Source: CAD feature listing. Evaluate the final solid. Frame: model axes, mm. Give positions to 0.01 mm unless a question says otherwise; leave off trailing zeros. Loops run counter-clockwise (first coordinate to the right, second up) from the corner with the lowest first, then second, coordinate; pieces in that order, holes last. Notation, with made-up numbers: (-39, 87) -> (-33, 87) arc R14 cw to (-33, 107) -> close; hole circle Ø6 at (25.25, -40). An arc over 180 degrees is marked (long way). Put each result on its own line as item: value.
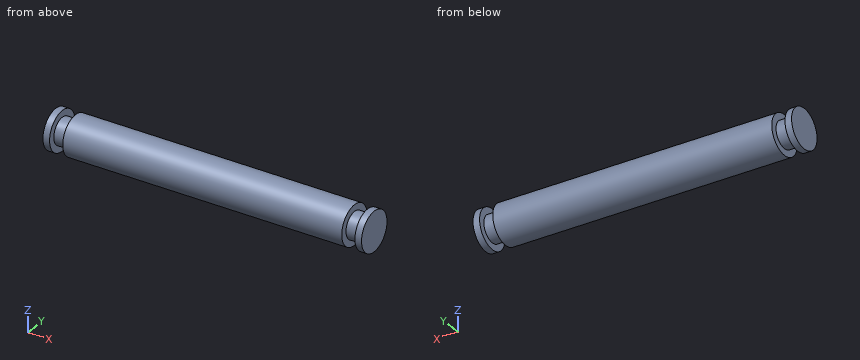
```python
from build123d import *

# Parameters (mm, degrees)
SKETCH_R     = 3
PAD_DEPTH    = 42.3
SKETCH001_R  = 2
PAD001_DEPTH = 2
SKETCH002_R  = 3
PAD002_DEPTH = 1
SKETCH003_R  = 2
PAD003_DEPTH = 2
SKETCH004_R  = 3
PAD004_DEPTH = 1


with BuildPart() as part:
    # Sketch → Pad (new body)
    with BuildSketch(Plane.YZ):
        Circle(SKETCH_R)
    extrude(amount=PAD_DEPTH)

    # Sketch001 (on Face3 of Pad) → Pad001 (join)
    with BuildSketch(Plane.YZ.offset(42.3)):
        Circle(SKETCH001_R)
    extrude(amount=PAD001_DEPTH)

    # Sketch002 (on Face5 of Pad001) → Pad002 (join)
    with BuildSketch(Plane.YZ.offset(44.3)):
        Circle(SKETCH002_R)
    extrude(amount=PAD002_DEPTH)

    # Sketch003 (on Face7 of Pad002) → Pad003 (join)
    with BuildSketch(Plane(origin=(0, 0, 0), x_dir=(0, 1, 0), z_dir=(-1, 0, 0))):
        Circle(SKETCH003_R)
    extrude(amount=PAD003_DEPTH)

    # Sketch004 (on Face9 of Pad003) → Pad004 (join)
    with BuildSketch(Plane(origin=(-2, 0, 0), x_dir=(0, 1, 0), z_dir=(-1, 0, 0))):
        Circle(SKETCH004_R)
    extrude(amount=PAD004_DEPTH)


solid = part.part
```
(1) Section D-D on z = 0.8. Return loops of the section in (x, y), then the cut area to 3 significant figures.
Calculated:
outline: (-3, -2.89) -> (-2, -2.89) -> (-2, -1.83) -> (0, -1.83) -> (0, -2.89) -> (42.3, -2.89) -> (42.3, -1.83) -> (44.3, -1.83) -> (44.3, -2.89) -> (45.3, -2.89) -> (45.3, 2.89) -> (44.3, 2.89) -> (44.3, 1.83) -> (42.3, 1.83) -> (42.3, 2.89) -> (0, 2.89) -> (0, 1.83) -> (-2, 1.83) -> (-2, 2.89) -> (-3, 2.89) -> close
area: 271 mm²
(2) Section A-A on z = -2.6. Return loops of the section in (x, y).
Calculated:
outline: (-3, -1.5) -> (-2, -1.5) -> (-2, 1.5) -> (-3, 1.5) -> close; (0, -1.5) -> (42.3, -1.5) -> (42.3, 1.5) -> (0, 1.5) -> close; (44.3, -1.5) -> (45.3, -1.5) -> (45.3, 1.5) -> (44.3, 1.5) -> close
(3) Section C-C on x = 8.5. Return loops of the section in (y, z).
Calculated:
outline: circle Ø6 at (0, 0)
(4) First-contact query: P1, Ø1.5, axis at x = 24, z = -1, coming from the -Y side. Flat tip, straight axial feed; report the tip coordinate or a pass-through.
Calculated:
P1: stops at y = -2.99
(5) Line query: probe 1 along X at (y, z) = (2.4, -0.25); probe 2 along Y at (x, z) = (41.5, -0.15); probe 3 along Z at (x, y) = (15, -1.9). Output: solid intervals per line, ascending. Write a range as from..to.
Calculated:
probe 1: x = -3..-2, 0..42.3, 44.3..45.3
probe 2: y = -3..3
probe 3: z = -2.32..2.32
(6) Section B-B on y = 0. Return loops of the section in (x, z).
Calculated:
outline: (-3, -3) -> (-2, -3) -> (-2, -2) -> (0, -2) -> (0, -3) -> (42.3, -3) -> (42.3, -2) -> (44.3, -2) -> (44.3, -3) -> (45.3, -3) -> (45.3, 3) -> (44.3, 3) -> (44.3, 2) -> (42.3, 2) -> (42.3, 3) -> (0, 3) -> (0, 2) -> (-2, 2) -> (-2, 3) -> (-3, 3) -> close
